Read the model definition and answer for the solid it produces. Units are mm, in the model's axes. A direction names the side the tool comes from. Coordinates: 2 decimals unless noted, no trailing zeros. Write each loop counter-clockwise with the first axis right and the second up, starting at its lowest first coordinate (ties: lowest second). Pieces come first, ordered by that corner, then holes. Notation, with made-up numbers: (-39, 0.5) -> (-15, 0.5) arc R19 cw to (-15, 7.5) -> close; hole circle Ø2 at (-21, 22). An arc over 180 degrees is marked (long way). Answer as a JSON object with one key per item and string values. Group by question number.
(1) For a pull along Y with two mould halves and no side action, classify faces 1 (the face through (-0.1, 17.3, 0)), 2 (the face through (-5.64, -18.9, -0.78)), 3 (the face through (7.91, -15.72, -0.78)), 4 (the face through (10.12, -14.22, -0.78)) as +Y half, -Y half, draft (parallel to the pull), parting line (faces both ways), or undercut.
(2) A flat-ended cylindrical pin translates along its axis: P1, Ø10, axis at x = 10.5, y = -3, coming from the -Z side. Find the tip coordinate at first contact, or state that the pin passes through.
(3) Find section B-B (x = 12). Give the vertices of the cut face in (y, z), then the cut area to 3 significant figures.
(4) Straight lines are drawn through the part: L1, parallel to X at y = 5, z = -0.95; L2, parallel to Y at x = -14.5, z = -0.4; L3, parallel to X at y = -7.5, z = -0.55. For each, find the intervals that lie inside material, in ascending order.
(5) Find section C-C (z = -1.15). Give the vertices of the cut face in (x, y).
(6) Which of the six approach directions +Z, -Z, +X, -X, +Y, -Y give full straight-line access (tool end or side, diameter ignored) to faces 5 (the face through (-0.1, 17.3, -1.588)), 6 (the face through (-5.257, -15.116, -0.783)), 7 (the face through (5.625, -18.863, -0.783))?
(7) Find section D-D (x = 3). Give the vertices of the cut face in (y, z), then the cut area to 3 significant figures.
(8) Find section A-A (y = 16). Give the vertices of the cut face in (x, z).
from build123d import *

# Parameters (mm, degrees)
F0_R     = 0.9906
F1_DEPTH = 1.5875


# Not quite as in the source:
# - ends of sketch curves that miss each other by under 0.0002 mm in the source are joined


with BuildPart() as f1:
    # F0 (on Top) → F1 (new body)
    with BuildSketch(Plane.XY):
        with BuildLine():
            Line((41.6924998, -18.8505592), (42.8484792, -21.3295484))
            ThreePointArc((42.8484792, -21.3295484), (36.6378236, 19.8468996), (30.4271688612, -21.32954561))
            Line((30.4271688612, -21.32954561), (31.5831474, -18.8505592))
            ThreePointArc((31.5831474, -18.8505592), (31.3595624423, -16.2949103348), (29.034512192, -15.2107228522))
            Line((29.034512192, -15.2107228522), (24.075517, -15.6445712))
            ThreePointArc((24.075517, -15.6445712), (36.6378236, 15.8590996), (49.2001483474, -15.6445903367))
            Line((49.2001483474, -15.6445903367), (44.2411358, -15.2107138))
            ThreePointArc((44.2411358, -15.2107138), (41.9160847577, -16.2949103348), (41.6924998, -18.8505592))
        make_face()
        with Locations((29.2581076, -17.7663602)):
            Circle(F0_R, mode=Mode.SUBTRACT)
        with Locations((44.0175396, -17.7663602)):
            Circle(F0_R, mode=Mode.SUBTRACT)
    extrude(amount=-F1_DEPTH)


with BuildPart() as f1_1:
    # F3: moved
    add(f1.part.moved(Location((-36.6378236, -19.8468996, 0))))


with BuildPart() as f1_2:
    # F4: moved
    add(f1_1.part.moved(Location((0, 21.0566, 0))))


solid = f1_2.part
Results below:
{
 "1": {"face 1": "draft", "face 2": "-Y half", "face 3": "undercut", "face 4": "undercut"},
 "2": {"P1": "passes through"},
 "3": {"outline": "(-17.3, -1.59) -> (-14.39, -1.59) -> (-14.39, 0) -> (-17.3, 0) -> close; (12.57, -1.59) -> (17.3, -1.59) -> (17.3, 0) -> (12.57, 0) -> close", "area": "12.1 mm2"},
 "4": {"L1": "x = -20.45 to -17.18, 17.18 to 20.45", "L2": "y = -15.27 to -12.28, 9.91 to 15.27", "L3": "x = -19.68 to -17.13, 17.13 to 19.68"},
 "5": {"outline": "(-12.56, -14.43) arc R18.26 cw (long way) to (12.56, -14.43) -> (7.6, -14) arc R2.57 ccw to (5.05, -17.64) -> (6.21, -20.12) arc R21.06 ccw (long way) to (-6.21, -20.12) -> (-5.05, -17.64) arc R2.57 ccw to (-7.6, -14) -> close; hole circle Ø1.98 at (-7.38, -16.56); hole circle Ø1.98 at (7.38, -16.56)"},
 "6": {"face 5": "-Z, +X, -X, +Y, -Y", "face 6": "+Z, -Z", "face 7": "+Z, -Z, -Y"},
 "7": {"outline": "(16.82, -1.59) -> (20.84, -1.59) -> (20.84, 0) -> (16.82, 0) -> close", "area": "6.38 mm2"},
 "8": {"outline": "(-13.69, -1.59) -> (-6.15, -1.59) -> (-6.15, 0) -> (-13.69, 0) -> close; (6.15, -1.59) -> (13.69, -1.59) -> (13.69, 0) -> (6.15, 0) -> close"}
}
